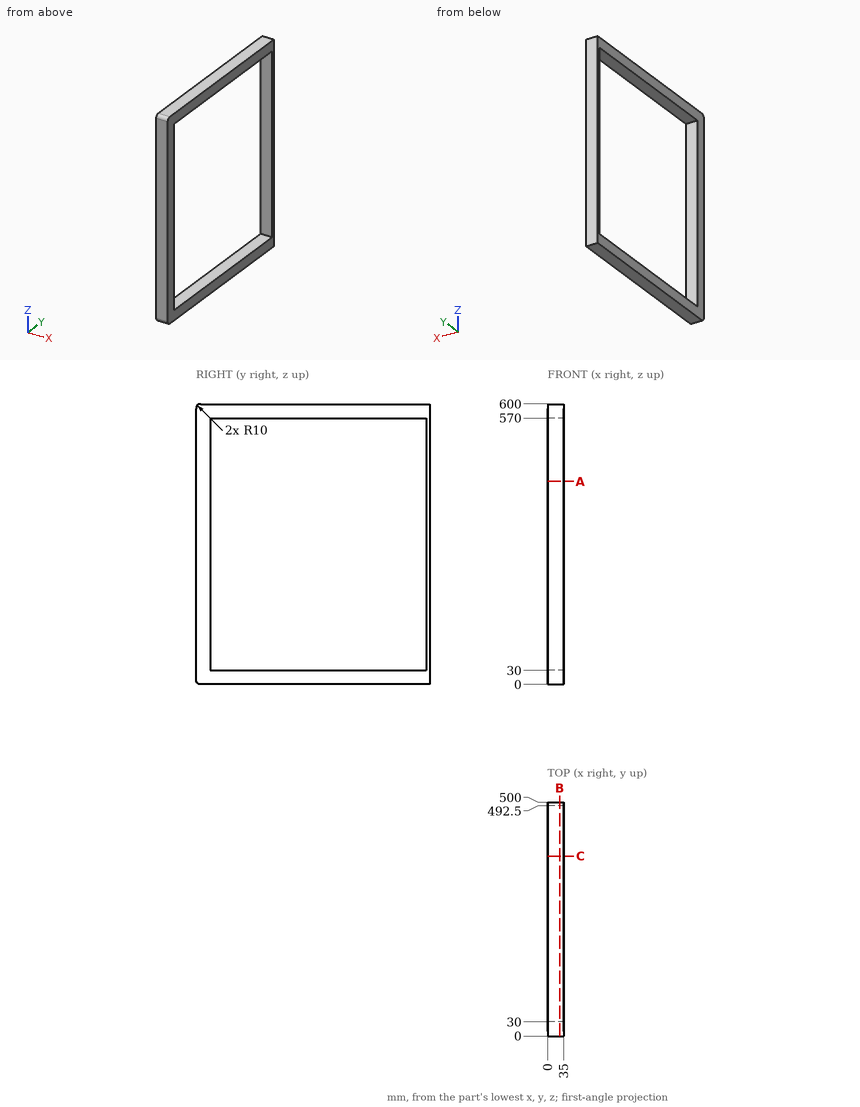
Input: dimensioned drawing with shaded views. Units: mm. Origin: part minimum x, y, z. Round coordinates to 2 decimals unless told otherwise and drop trailing zeros. Loops run counter-clockwise (first coordinate to the right, second up) from the corner with the lowest first, then second, coordinate; pieces in that order, holes last. Notation, with made-up numbers: M 40,33 L 80,33 A33 ccw 80,71 Z; hole C 10,34 d2. An arc over 180 degrees is marked long. Answer in a Markdown table with one row per item. Add a question column.
1. Section C-C (y = 385). Output: boundary loops of the cut face in (x, z), and give its area (3 significant figures).
2. Section A-A (z = 434.5). Output: boundary loops of the cut face in (x, y), and give its area (3 significant figures).
3. Ray query, probe 1 along Z at (x, y) = (29.5, 466); probe 2 along Y at (x, z) = (9, 566.5). Return the intervals inside material, ascending.
4. Section B-B (x = 25.5). Output: boundary loops of the cut face in (y, z), and give its area (3 significant figures).
Values follow:
| question | item | result |
|---|---|---|
| 1 | outline | M 0,0 L 35,0 L 35,30 L 0,30 Z; M 0,570 L 35,570 L 35,600 L 0,600 Z |
| 1 | area | 2,100 mm^2 |
| 2 | outline | M 0,0 L 35,0 L 35,30 L 0,30 Z; M 0,492.5 L 35,492.5 L 35,500 L 0,500 Z |
| 2 | area | 1,310 mm^2 |
| 3 | probe 1 | 0 to 30, 570 to 600 |
| 3 | probe 2 | 0 to 30, 492.5 to 500 |
| 4 | outline | M 0,10 A10 ccw 10,0 L 500,0 L 500,600 L 10,600 A10 ccw 0,590 Z; hole M 30,30 L 492.5,30 L 492.5,570 L 30,570 Z |
| 4 | area | 50,200 mm^2 |
